Can you work these out from the model? Positions are in its coordinate system, mm. Face numbers are marked on the shaded views. A direction names the side the tool comes from. Round coordinates to 2 decimals unless told otherwise and drop trailing zeros. Order: outer loops, then holes, each group sorted by start corner. A loop starts at its lowest first (then second) coordinate and runs counter-clockwise, first axis right, second up.
Q1. If we section it at C-C (y = -5.5): Please give me the cut outline in (x, z), plus the area to 3 significant figures.
Q2. If we section it at B-B (z = -2.25): Please give me the cut outline in (x, y).
Q3. Will these pins go through, and if not, where does the flat tip stop? P1, Ø5, axis at x = -17.85, y = 0, coming from the -Z side; P2, Ø1, axis at y = 7.5, z = 11, coming from the +X side; P3, Ø0.6, axis at y = 8, z = 10.5, coming from the -X side.
Q4. If I drill on line 1 (X direction, y = 0, z = 9.75); line 2 (X direction, y = 0, z = 6.75); line 3 (X direction, y = 10, z = 11.25), over which ranges is the centre line in solid material (lowest first)?
Q5. If we section it at D-D (x = -28): Please give me the cut outline in (y, z).
Q6. We'd pull the mould along X, two halves only. Please class the marked faces 1, 2 and 3: pulls with the +X half, pulls with the -X half, needs draft (parallel to the pull), parting line crosses it, or undercut.
Q7. If we section it at A-A (x = 3): Please give me the cut outline in (y, z), plus the area to 3 significant figures.
Q8. For the marked faces 4, 5, 6, 7 and 8, which set-ups out of +Z, -Z, +X, -X, +Y, -Y let a thin tool reach every point of the face, with its end or its side?
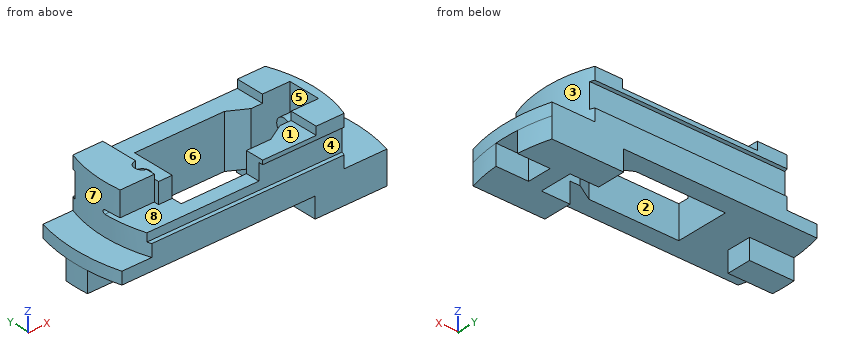
from build123d import *

# Parameters (mm, degrees)
F1_DEPTH      = 3
F3_DEPTH      = 5
F5_DEPTH      = 3.001
F7_DEPTH      = 12
F8_W          = 1
F8_H          = 6
F9_DEPTH      = 34.001
F9_DEPTH_BACK = 34.001
F10_R         = 1.85
F11_DEPTH     = 7.5
F13_DEPTH     = 2
F14_DEPTH     = 7
F18_DEPTH     = 16.65
F19_R         = 2
F20_DEPTH     = 5


with BuildPart() as f1:
    # F0 (on Top) → F1 (new body)
    with BuildSketch(Plane.XY):
        with BuildLine():
            ThreePointArc((32.5, -11), (34, 0), (32.5, 11))
            Line((32.5, 11), (-32.5, 11))
            ThreePointArc((-32.5, 11), (-34, 0), (-32.5, -11))
            Line((-32.5, -11), (32.5, -11))
        make_face()
    extrude(amount=-F1_DEPTH)

    # F2 (on face) → F3 (join)
    with BuildSketch(Plane(origin=(0, 0, -3), x_dir=(1, 0, 0), z_dir=(0, 0, -1))):
        with BuildLine():
            Line((-23, 3), (-33.8903201257, 3))
            ThreePointArc((-33.8903201257, 3), (-34, 0), (-33.8903201257, -3))
            Line((-33.8903201257, -3), (-23, -3))
            Line((-23, -3), (-23, 0))
            Line((-23, 0), (-23, 3))
        make_face()
        with BuildLine():
            Line((25.8903201257, 3), (33.8903201257, 3))
            ThreePointArc((33.8903201257, 3), (33.3932899234, 7.0344329916), (32.5, 11))
            Line((32.5, 11), (14.8903201257, 11))
            Line((14.8903201257, 11), (14.8903201257, 4))
            Line((14.8903201257, 4), (21.8903201257, 4))
            Line((21.8903201257, 4), (21.8903201257, 0))
            Line((21.8903201257, 0), (21.8903201257, -4))
            Line((21.8903201257, -4), (14.8903201257, -4))
            Line((14.8903201257, -4), (14.8903201257, -11))
            Line((14.8903201257, -11), (32.5, -11))
            ThreePointArc((32.5, -11), (33.3932899234, -7.0344329916), (33.8903201257, -3))
            Line((33.8903201257, -3), (25.8903201257, -3))
            Line((25.8903201257, -3), (25.8903201257, 0))
            Line((25.8903201257, 0), (25.8903201257, 3))
        make_face()
    extrude(amount=F3_DEPTH)

    # F4 (on face) → F5 (cut, through all)
    with BuildSketch(Plane(origin=(0, 0, -3), x_dir=(1, 0, 0), z_dir=(0, 0, -1))):
        Polygon((21.8903201257, -4), (21.8903201257, 4), (14.8903201257, 4), (12.3903201257, 4), (8, 6.5), (-14, 6.5), (-14, 0), (-14, -6.5), (8, -6.5), (12.3903201257, -4), (14.8903201257, -4), align=None)
    extrude(amount=-F5_DEPTH, mode=Mode.SUBTRACT)

    # F6 (on face) → F7 (join)
    with BuildSketch(Plane.XY):
        with BuildLine():
            Line((21.9885364227, 11), (-25.1761398662, 11))
            ThreePointArc((-25.1761398662, 11), (-27, 0), (-25.1761398662, -11))
            Line((-25.1761398662, -11), (21.9885364227, -11))
            ThreePointArc((21.9885364227, -11), (24, 0), (21.9885364227, 11))
        make_face()
        Polygon((12.3903201257, 4), (21.8903201257, 4), (21.8903201257, -4), (12.3903201257, -4), (8, -6.5), (-14, -6.5), (-14, 6.5), (8, 6.5), align=None, mode=Mode.SUBTRACT)
    extrude(amount=F7_DEPTH)

    # F8 (on Right) → F9 (cut, two sides)
    with BuildSketch(Plane.YZ) as f9_sk:
        with Locations((-10.5, 6)):
            Rectangle(F8_W, F8_H)
        with Locations((10.5, 6)):
            Rectangle(F8_W, F8_H)
    extrude(amount=-F9_DEPTH, mode=Mode.SUBTRACT)
    extrude(f9_sk.sketch, amount=F9_DEPTH_BACK, mode=Mode.SUBTRACT)

    # F10 (on face) → F11 (cut)
    with BuildSketch(Plane.XY.offset(12)):
        with Locations((-17.85, 0)):
            Circle(F10_R)
    extrude(amount=-F11_DEPTH, mode=Mode.SUBTRACT)

    # F12 (on face) → F13 (cut)
    with BuildSketch(Plane.XY.offset(12)):
        with BuildLine():
            Line((15.15, 11), (-17.85, 11))
            Line((-17.85, 11), (-17.85, 1.85))
            ThreePointArc((-17.85, 1.85), (-16.5418524548, 1.3081475452), (-16, 0))
            ThreePointArc((-16, 0), (-16.3756357302, -1.1174748319), (-17.35, -1.7811513131))
            Line((-17.35, -1.7811513131), (-17.35, -4))
            Line((-17.35, -4), (-14, -4))
            Line((-14, -4), (-14, 6.5))
            Line((-14, 6.5), (8, 6.5))
            Line((8, 6.5), (12.3903201257, 4))
            Line((12.3903201257, 4), (15.15, 4))
            Line((15.15, 4), (15.15, 11))
        make_face()
        Polygon((-17.35, -4), (-17.85, -4), (-17.85, -11), (2, -11), (2, -6.5), (-14, -6.5), (-14, -4), align=None)
        Polygon((15.15, -11), (15.15, -4), (12.3903201257, -4), (8, -6.5), (2, -6.5), (2, -11), align=None)
    extrude(amount=-F13_DEPTH, mode=Mode.SUBTRACT)

    # F12 (on face) → F14 (cut)
    with BuildSketch(Plane.XY.offset(12)):
        Polygon((-17.35, -4), (-17.85, -4), (-17.85, -11), (2, -11), (2, -6.5), (-14, -6.5), (-14, -4), align=None)
        with BuildLine():
            Line((-18.35, -4), (-26.7644673502, -4))
            ThreePointArc((-26.7644673502, -4), (-26.1550919462, -7.5419291994), (-25.1761398662, -11))
            Line((-25.1761398662, -11), (-17.85, -11))
            Line((-17.85, -11), (-17.85, -4))
            Line((-17.85, -4), (-18.35, -4))
        make_face()
        with BuildLine():
            ThreePointArc((-17.35, -1.7811513131), (-17.5976410584, -1.8327070046), (-17.85, -1.85))
            Line((-17.85, -1.85), (-17.85, -4))
            Line((-17.85, -4), (-17.35, -4))
            Line((-17.35, -4), (-17.35, -1.7811513131))
        make_face()
        with BuildLine():
            ThreePointArc((-17.85, -1.85), (-18.1023589416, -1.8327070046), (-18.35, -1.7811513131))
            Line((-18.35, -1.7811513131), (-18.35, -4))
            Line((-18.35, -4), (-17.85, -4))
            Line((-17.85, -4), (-17.85, -1.85))
        make_face()
    extrude(amount=-F14_DEPTH, mode=Mode.SUBTRACT)

    # F17 (on plane+point) → F18 (cut, through all)
    with BuildSketch(Plane.YZ.offset(-34)):
        with BuildLine():
            Line((-4, 6), (-4, 5))
            Line((-4, 5), (0, 5))
            ThreePointArc((0, 5), (0.5, 5.5), (0, 6))
            Line((0, 6), (-4, 6))
        make_face()
    extrude(amount=F18_DEPTH, mode=Mode.SUBTRACT)

    # F19 (on face) → F20 (join)
    with BuildSketch(Plane(origin=(21.8903201257, 0, 0), x_dir=(0, -1, 0), z_dir=(-1, 0, 0))):
        with Locations((0, 6)):
            Circle(F19_R)
    extrude(amount=F20_DEPTH)


solid = f1.part
Solution:
1. outline: (-33.63, -3) - (-14, -3) - (-14, 5) - (-26.55, 5) - (-26.55, 0) - (-33.63, 0) - close; (9.76, -3) - (14.89, -3) - (14.89, -8) - (33.63, -8) - (33.63, 0) - (23.51, 0) - (23.51, 12) - (15.15, 12) - (15.15, 10) - (9.76, 10) - close
1. area: 441 mm2
2. outline: (-32.5, -11) - (32.5, -11) arc R41.08 ccw to (32.5, 11) - (-32.5, 11) arc R41.08 ccw to start; hole (-14, -6.5) - (8, -6.5) - (12.39, -4) - (21.89, -4) - (21.89, 4) - (12.39, 4) - (8, 6.5) - (-14, 6.5) - close
3. P1: stops at z = -3
3. P2: stops at x = 23.2
3. P3: stops at x = -26.12
4. line 1: x = -27 to -19.7, -16 to -14, 21.89 to 24
4. line 2: x = -27 to -19.7, -16 to -14, 16.89 to 24
4. line 3: x = -25.5 to -17.85, 15.15 to 22.35
5. outline: (-11, -3) - (-3, -3) - (-3, -8) - (3, -8) - (3, -3) - (11, -3) - (11, 0) - (-11, 0) - close
6. face 1: needs draft
6. face 2: undercut
6. face 3: pulls with the +X half
7. outline: (-11, -3) - (-6.5, -3) - (-6.5, 10) - (-11, 10) - (-11, 9) - (-10, 9) - (-10, 3) - (-11, 3) - close; (6.5, -3) - (11, -3) - (11, 3) - (10, 3) - (10, 9) - (11, 9) - (11, 10) - (6.5, 10) - close
7. area: 105 mm2
8. face 4: +X, -X, -Y
8. face 5: none
8. face 6: +Z, -Z
8. face 7: +Z, -X
8. face 8: -X, -Y
